Geometry: final body of the model. Coordinates: model frame, mm. Face numbers are marked on the shaded views. Give positions to 0.01 mm unless a question says otherwise; leave off trailing zeros. Write each loop counter-clockwise with the first axis right and the second up, starting at its lowest first coordinate (ties: lowest second). Pieces come first, ordered by that corner, then holes. Notation, with made-up numbers: (-28, 67) -> (-17, 67) arc R26 ccw to (-17, 95) -> close; hole circle Ø9 at (-19.75, 86). An arc over 180 degrees is marked (long way). Answer as a JSON object with one key per item and string values.
from build123d import *

# Parameters (mm, degrees)
SKETCH_1_R               = 21
SKETCH_1_R_2             = 10
EXTRUDE_1_DEPTH          = 45
SKETCH_4_R               = 21
SKETCH_4_R_2             = 10
EXTRUDE_2_DEPTH          = 85
CUT_EXTRUDE_3_DEPTH      = 15
CUT_EXTRUDE_START        = -15
CUT_EXTRUDE_4_DEPTH      = 15
CUT_EXTRUDE_6_DEPTH      = 25
CUT_EXTRUDE_START_2      = 20.4
CUT_EXTRUDE_7_DEPTH      = 2.45
PATTERN_CIRCULAR_1_COUNT = 4
SKETCH_14_R              = 1.6
CUT_EXTRUDE_8_DEPTH      = 22.45
PATTERN_CIRCULAR_2_COUNT = 4


with BuildPart() as part:
    # 草图1 → 凸台-拉伸1 (new body)
    with BuildSketch(Plane(origin=(0, 0, 0), x_dir=(1, 0, 0), z_dir=(0, 1, 0))):
        with Locations(Location((0, 0, 0), (0, 0, 90))):
            Circle(SKETCH_1_R)
        with Locations(Location((0, 0, 0), (0, 0, 90))):
            Circle(SKETCH_1_R_2, mode=Mode.SUBTRACT)
    extrude(amount=EXTRUDE_1_DEPTH)

    # 草图4 → 凸台-拉伸2 (add)
    with BuildSketch(Plane(origin=(0, 45, 0), x_dir=(1, 0, 0), z_dir=(0, 1, 0))):
        with Locations(Location((0, 0, 0), (0, 0, 90))):
            Circle(SKETCH_4_R)
        with Locations(Location((0, 0, 0), (0, 0, 90))):
            Circle(SKETCH_4_R_2, mode=Mode.SUBTRACT)
    extrude(amount=EXTRUDE_2_DEPTH)

    # 草图11 → 切除-拉伸3 (cut)
    with BuildSketch(Plane(origin=(0, 0, 0), x_dir=(1, 0, 0), z_dir=(0, 1, 0))):
        with BuildLine():
            Line((-20.396078054, 5), (-20.396078054, -5))
            ThreePointArc((-20.396078054, -5), (-21, 0), (-20.396078054, 5))
        make_face()
        with BuildLine():
            Line((-5, -20.396078054), (5, -20.396078054))
            ThreePointArc((5, -20.396078054), (0, -21), (-5, -20.396078054))
        make_face()
        with BuildLine():
            Line((20.396078054, -5), (20.396078054, 5))
            ThreePointArc((20.396078054, 5), (21, 0), (20.396078054, -5))
        make_face()
        with BuildLine():
            Line((5, 20.396078054), (-5, 20.396078054))
            ThreePointArc((-5, 20.396078054), (0, 21), (5, 20.396078054))
        make_face()
    extrude(amount=CUT_EXTRUDE_3_DEPTH, mode=Mode.SUBTRACT)

    # 草图5 → 切除-拉伸4 (cut)
    with BuildSketch(Plane(origin=(0, 130, 0), x_dir=(1, 0, 0), z_dir=(0, 1, 0)).offset(CUT_EXTRUDE_START)):
        with BuildLine():
            Line((-20.396078054, 5), (-20.396078054, -5))
            ThreePointArc((-20.396078054, -5), (-21, 0), (-20.396078054, 5))
        make_face()
        with BuildLine():
            Line((-5, -20.396078054), (5, -20.396078054))
            ThreePointArc((5, -20.396078054), (0, -21), (-5, -20.396078054))
        make_face()
        with BuildLine():
            Line((20.396078054, -5), (20.396078054, 5))
            ThreePointArc((20.396078054, 5), (21, 0), (20.396078054, -5))
        make_face()
        with BuildLine():
            Line((5, 20.396078054), (-5, 20.396078054))
            ThreePointArc((-5, 20.396078054), (0, 21), (5, 20.396078054))
        make_face()
    extrude(amount=CUT_EXTRUDE_4_DEPTH, mode=Mode.SUBTRACT)

    # 草图12 → 切除-拉伸6 (cut)
    with BuildSketch(Plane.XY):
        Polygon((0, 110), (8, 110), (8, 102), (-8, 102), (-8, 110), align=None)
    extrude(amount=CUT_EXTRUDE_6_DEPTH, mode=Mode.SUBTRACT)

    # 草图13 → 切除-拉伸7 (cut)
    with BuildSketch(Plane(origin=(0, 0, 0), x_dir=(0, 0, -1), z_dir=(1, 0, 0)).offset(CUT_EXTRUDE_START_2)):
        Polygon((0, 128.233161507), (-2.8, 126.616580754), (-2.8, 123.383419246), (0, 121.766838493), (2.8, 123.383419246), (2.8, 126.616580754), align=None)
        Polygon((0, 8.233161507), (-2.8, 6.616580754), (-2.8, 3.383419246), (0, 1.766838493), (2.8, 3.383419246), (2.8, 6.616580754), align=None)
    cut_extrude_7 = extrude(amount=-CUT_EXTRUDE_7_DEPTH, mode=Mode.SUBTRACT)

    # 阵列(圆周)1: 切除-拉伸7 ×4 about axis
    pattern_circular_1_axis = Axis((0, 0, 0), (0, 1, 0))
    for i in range(1, PATTERN_CIRCULAR_1_COUNT):
        add(cut_extrude_7.rotate(pattern_circular_1_axis, i * 360 / PATTERN_CIRCULAR_1_COUNT), mode=Mode.SUBTRACT)

    # 草图14 → 切除-拉伸8 (cut)
    with BuildSketch(Plane(origin=(0, 0, 0), x_dir=(0, 0, -1), z_dir=(1, 0, 0))):
        with Locations(Location((0, 125, 0), (0, 0, 180))):
            Circle(SKETCH_14_R)
        with Locations(Location((0, 5, 0), (0, 0, 180))):
            Circle(SKETCH_14_R)
    cut_extrude_8 = extrude(amount=CUT_EXTRUDE_8_DEPTH, mode=Mode.SUBTRACT)

    # 阵列(圆周)2: 切除-拉伸8 ×4 about axis
    pattern_circular_2_axis = Axis((0, 45, 0), (0, -1, 0))
    for i in range(1, PATTERN_CIRCULAR_2_COUNT):
        add(cut_extrude_8.rotate(pattern_circular_2_axis, i * 360 / PATTERN_CIRCULAR_2_COUNT), mode=Mode.SUBTRACT)


solid = part.part
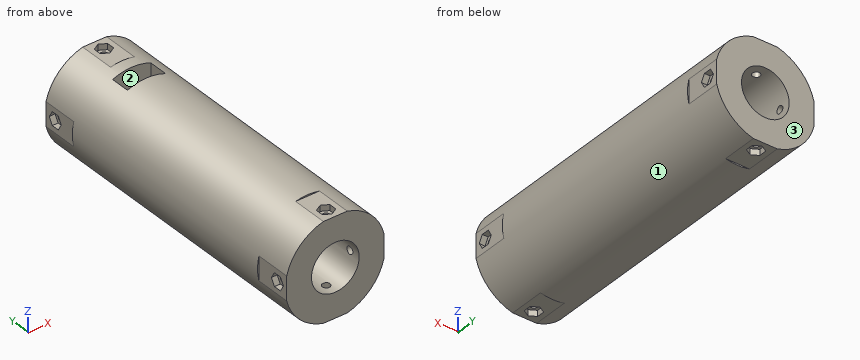
Q1. Cut plane B-B (y = 27). Return the cut outline in (x, z).
Values:
{"outline": "circle Ø42 at (0, 0); hole circle Ø20 at (0, 0)"}
Q2. Mould query, pull axis X, two halves, no side actions, for the marked faces 1, 2 and 3. Classes: pulls with the +X half, pulls with the -X half, needs draft (parallel to the pull), parting line crosses it, or undercut.
Values:
{"face 1": "parting line crosses it", "face 2": "undercut", "face 3": "needs draft"}
Q3. Cut plane C-C (x = 15). Return the cut outline in (y, z), and give its area (3 significant figures).
Values:
{"outline": "(0, -14.7) -> (130, -14.7) -> (130, 14.7) -> (0, 14.7) -> close; hole circle Ø3.2 at (5, 0); hole circle Ø3.2 at (125, 0)", "area": "3,810 mm²"}
Q4. Material intervals for L1, parallel to Y at x = -13.25, z = 0; L2, parallel to Y at x = 0, z = 14; L3, parallel to X at y = 74, z = 0, sorted ascending. Write a range as from..to.
Values:
{"L1": "0..3.4, 6.6..123.4, 126.6..130", "L2": "0..3.4, 6.6..102, 110..123.4, 126.6..130", "L3": "-21..-10, 10..21"}
Q5. Cut plane D-D (y = 125). State how many separate pieces and enclosed holes the cut face has, and give its area (3 significant figures).
Values:
{"separate pieces": "4", "enclosed holes": "0", "area": "898 mm²"}
Q6. First-contact query: P1, Ø12, axis at y = 67, z = -9.5, coming from the -X side; P2, Ø2.5, axis at y = 5, z = -19.5, coming from the +X side; P3, Ø3.5, axis at y = 5, z = 0, coming from the -X side. Flat tips, straight axial feed; report the tip coordinate or a pass-through.
Values:
{"P1": "x = -20.71", "P2": "x = 10.39", "P3": "x = -17.95"}
Q7. Cut plane A-A (z = 16.5). Return the cut outline in (x, y).
Values:
{"outline": "(-12.99, 0) -> (12.99, 0) -> (12.99, 130) -> (-12.99, 130) -> close; hole (-8, 102) -> (8, 102) -> (8, 110) -> (-8, 110) -> close; hole circle Ø3.2 at (0, 5); hole circle Ø3.2 at (0, 125)"}
